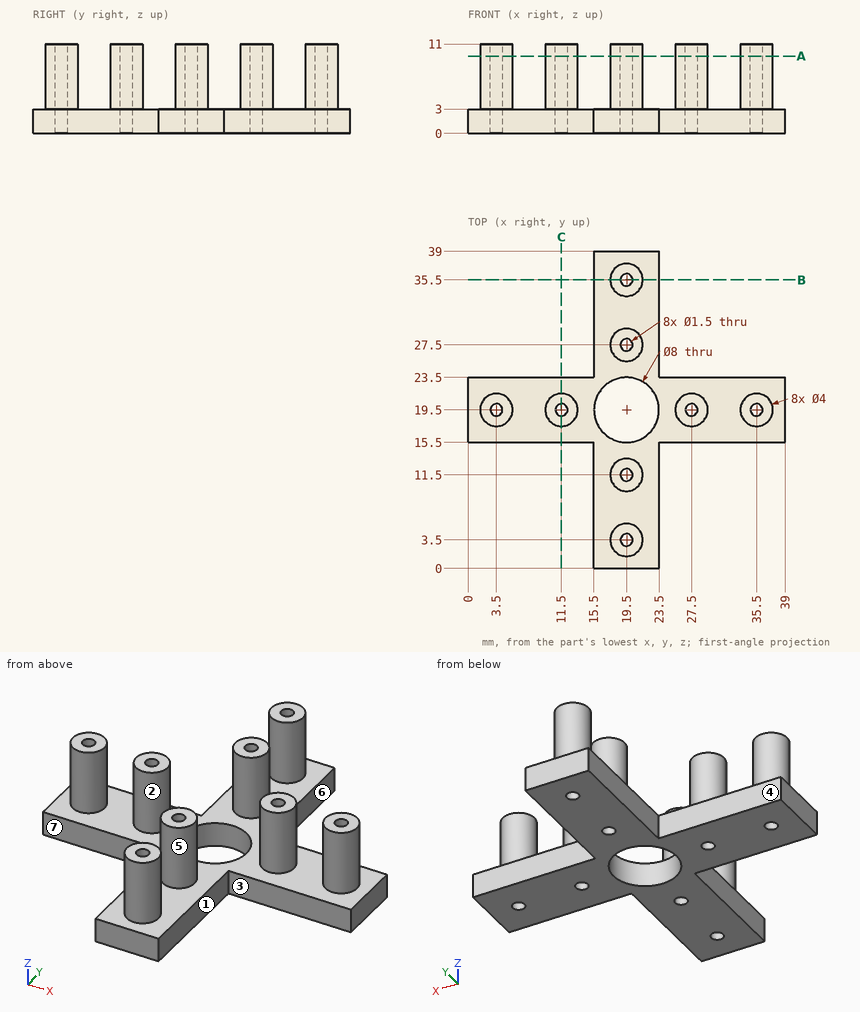
Part print with two shaded views. Sizes in mm from the minimum x, y, z corner. A direction names the side the tool comes from. Coordinates: 2 decimals unless noted, no trailing zeros. Order: outer loops, then holes, each group sorted by start corner. A loop starts at its lowest first (then second) coordinate and runs counter-clockwise, first axis right, second up. Notation, with made-up numbers: M 76,54 L 133,54 A21 cw 133,64 Z; hole C 5.25,58.25 d2. An arc over 180 degrees is marked long. Use a Markdown table: item, result.
(1) Cut at B-B on y = 35.5. Write the cut outline in (x, z), then the cut area to 3 significant figures.
A:
| item | result |
|---|---|
| outline | M 15.5,0 L 18.75,0 L 18.75,11 L 17.5,11 L 17.5,3 L 15.5,3 Z; M 20.25,0 L 23.5,0 L 23.5,3 L 21.5,3 L 21.5,11 L 20.25,11 Z |
| area | 39.5 mm^2 |
(2) Probe L1, parallel to Y at x = 19.5, z = 2.05; L2, parallel to Z at x = 15, y = 17; L3, parallel to X at y = 15, z = 2.75. List the from-to ranges inside material, lowest first.
A:
| item | result |
|---|---|
| L1 | y = 0 to 2.75, 4.25 to 10.75, 12.25 to 15.5, 23.5 to 26.75, 28.25 to 34.75, 36.25 to 39 |
| L2 | z = 0 to 3 |
| L3 | x = 15.5 to 23.5 |
(3) Pull direction X, two halves, no side cores. Call the marked faces 1, 2 and 3: released by +X, released by -X, zero draft, split by the parting line, or undercut.
A:
| item | result |
|---|---|
| face 1 | released by +X |
| face 2 | undercut |
| face 3 | zero draft |
(4) Cut at A-A on z = 9.5. State how many separate pieces and enclosed holes the cut face has, then the cut area to 3 significant figures.
A:
| item | result |
|---|---|
| separate pieces | 8 |
| enclosed holes | 8 |
| area | 86.4 mm^2 |
(5) Flat gauge pins, fed straight in: pin 1 (2.5 mm diameter, centred on y = 9, z = 2, fed in from -X); pin 2 (3 mm diameter, centred on y = 8.5, z = 6.5, fed in from +X); pin 3 (0.9 mm diameter, centred on x = 4.5, z = 2, fed in from -Y); pin 4 (1.4 mm diameter, centred on x = 19.5, y = 27.5, fed in from +Z). Where does each tip first touch, or does it go through?
A:
| item | result |
|---|---|
| pin 1 | stops at x = 15.5 |
| pin 2 | stops at x = 20.82 |
| pin 3 | stops at y = 15.5 |
| pin 4 | passes through |
(6) Tool access for the marked faces 4, 5, 6 and 7: list every direction of +Z, -Z, +X, -X, +Y, -Y with a clear straight run to the whole face (end or side of a thin tool).
A:
| item | result |
|---|---|
| face 4 | +Z, -Z, -X, +Y |
| face 5 | +Z |
| face 6 | +Z, -Z, +X, +Y |
| face 7 | +Z, -Z, -X, -Y |
